Work out the finished part from the listing and answer in its coordinate system (mm). A direction names the side the tool comes from. Round coordinates to 2 decimals unless told otherwise and drop trailing zeros. Loops run counter-clockwise (first coordinate to the right, second up) from the corner with the lowest first, then second, coordinate; pieces in that order, holes last. Notation, with made-up numbers: (10.25, 57) -> (45.25, 57) arc R30 cw to (45.25, 81) -> close; hole circle Ø6 at (15, 60.5). An arc over 180 degrees is marked (long way). Write item = value, one per line. Start each with the question number.
```python
from build123d import *

# Parameters (mm, degrees)
BOSS_EXTRUDE1_DEPTH             = 50
BOSS_EXTRUDE2_START             = 13.15
BOSS_EXTRUDE2_DEPTH             = 13.15
BOSS_EXTRUDE3_DEPTH             = 21.75
BOSS_EXTRUDE3_DEPTH_BACK        = 63.15
CUT_EXTRUDE1_DEPTH              = 145.663436984
FILLET1_R                       = 3
CUT_EXTRUDE2_DEPTH              = 129.082637169
TAP_DRILL_FOR_M4X0_7_TAP1_D     = 3.3
TAP_DRILL_FOR_M4X0_7_TAP1_DEPTH = 10
TAP_DRILL_FOR_M4X0_7_TAP1_TIP   = 0.991420021


with BuildPart() as part:
    # Sketch1 → Boss-Extrude1 (new body)
    with BuildSketch(Plane.XY):
        with BuildLine():
            Line((36, 0), (63.5, 0))
            ThreePointArc((63.5, 0), (49.923691771, -39.241241061), (15, -61.702917273))
            Line((15, -61.702917273), (15, -32.726136344))
            ThreePointArc((15, -32.726136344), (30.298514815, -19.442222095), (36, 0))
        make_face()
    extrude(amount=BOSS_EXTRUDE1_DEPTH)

    # Sketch2 → Boss-Extrude2 (add)
    with BuildSketch(Plane(origin=(0, 0, 0), x_dir=(-1, 0, 0), z_dir=(0, 0, -1)).offset(BOSS_EXTRUDE2_START)):
        with BuildLine():
            Line((-45, 0), (-63.5, 0))
            ThreePointArc((-63.5, 0), (-49.923691771, -39.241241061), (-15, -61.702917273))
            Line((-15, -61.702917273), (-15, -42.426406871))
            ThreePointArc((-15, -42.426406871), (-36.742346142, -25.980762114), (-45, 0))
        make_face()
    extrude(amount=-BOSS_EXTRUDE2_DEPTH)

    # Sketch3 → Boss-Extrude3 (add, two sides: drawn at the far end of the back side and taken through both)
    with BuildSketch(Plane(origin=(0, 0, -13.15), x_dir=(-1, 0, 0), z_dir=(0, 0, -1)).offset(-BOSS_EXTRUDE3_DEPTH_BACK)):
        with BuildLine():
            Line((-63.5, 0), (-83.5, 0))
            ThreePointArc((-83.5, 0), (-64.127802083, -53.477799132), (-15, -82.141645954))
            Line((-15, -82.141645954), (-15, -61.702917273))
            ThreePointArc((-15, -61.702917273), (-49.923691771, -39.241241061), (-63.5, 0))
        make_face()
    extrude(amount=BOSS_EXTRUDE3_DEPTH + BOSS_EXTRUDE3_DEPTH_BACK)

    # Sketch4 → Cut-Extrude1 (cut, through all)
    with BuildSketch(Plane.XY.offset(50)):
        with BuildLine():
            Line((15, -32.726136344), (68.901001848, -47.16886626))
            ThreePointArc((68.901001848, -47.16886626), (45.449074332, -70.047352857), (15, -82.141645954))
            Line((15, -82.141645954), (15, -32.726136344))
        make_face()
    extrude(amount=-CUT_EXTRUDE1_DEPTH, mode=Mode.SUBTRACT)

    # Fillet1
    fillet1_edges = [part.edges().sort_by_distance(p)[0] for p in [
        (36, 0, 25),
        (15, -32.726136344, 25),
    ]]
    fillet(fillet1_edges, radius=FILLET1_R)

    # Sketch5 → Cut-Extrude2 (cut, through all)
    with BuildSketch(Plane.XY.offset(50)):
        with BuildLine():
            Line((83.5, 0), (68.901001848, -47.16886626))
            ThreePointArc((68.901001848, -47.16886626), (79.766796521, -24.688219313), (83.5, 0))
        make_face()
    extrude(amount=-CUT_EXTRUDE2_DEPTH, mode=Mode.SUBTRACT)

    # Tap Drill for M4x0.7 Tap1
    with Locations(Plane(origin=(76.200500924, -23.58443313, 0), x_dir=(0, 0, -1), z_dir=(0.9552909762953877, -0.29566729715781054, 0))):
        with Locations((-35, 15), (-35, -15), (-5, 15), (-5, -15)):
            Hole(TAP_DRILL_FOR_M4X0_7_TAP1_D / 2, depth=TAP_DRILL_FOR_M4X0_7_TAP1_DEPTH)
            with Locations((0, 0, -(TAP_DRILL_FOR_M4X0_7_TAP1_DEPTH + TAP_DRILL_FOR_M4X0_7_TAP1_TIP / 2))):  # 118° drill point
                Cone(0, TAP_DRILL_FOR_M4X0_7_TAP1_D / 2, TAP_DRILL_FOR_M4X0_7_TAP1_TIP, mode=Mode.SUBTRACT)


solid = part.part
```
Item 1: Find the intervals of material crossed by line 1 along Z through (x, y) = (61.5, -3); line 2 along Y through (x, z) = (49.5, 22.5); line 3 along X through (y, z) = (-28, 40), in increasing order. Write a range as [from, to].
Item 2: Section A-A (z = 8) is taken. Determine the outline of the cut face in (x, y).
Item 3: The mould has two halves that part along X. Classify faces 4 (the flat face through (61, 0, 18)), 5 (the cylindrical face through (66.94, -36.35, 33.35)), 6 (the cylindrical face through (59.388, -22.479, -23.873)): pulls with the +X half, pulls with the -X half, needs draft (parallel to the pull), parting line crosses it, or undercut.
Item 4: Section D-D (y = -22) is taken. Determine the outline of the cut face in (x, z).
Item 5: A tool of negligible diameter and unlimited length cuts with its end or side. For faces 1 (the cylindrical face through (40.134, -20.353, -6.667)), 2 (the cylindrical face through (31.261, -17.853, 24.65)), 3 (the conical face through (70.304, -6.044, 35.286)), from which of +Z, -Z, +X, -X, +Y, -Y can it reach the whole face along a straight path? Write none if from no direction.
Item 6: Flat-ended cylindrical pins translate along their axes: pin 1 (1.5 mm diameter, centred on x = 50, y = -15, fed in from -Z); pin 2 (6 mm diameter, centred on y = -38, z = 27.5, fed in from +X); pin 3 (3 mm diameter, centred on y = -26.5, z = -13.5, fed in from -X); pin 4 (11 mm diameter, centred on x = 53, y = -31, fed in from -Z). Find the tip coordinate at first contact, or state that the pin passes through.
Item 7: Section C-C (x = 31) is taken. Determine the outline of the cut face in (y, z), then the cut area to 3 significant figures.
Item 8: Section B-B (y = -31) is taken. Determine the outline of the cut face in (x, z), then the cut area to 3 significant figures.
Worked answers:
q1.line_1 = [-13.15, 50]
q1.line_2 = [-41.97, 0]
q1.line_3 = [22.63, 74.83]
q2.outline = (20.98, -29.25) arc R3 ccw to (21.95, -34.59) -> (68.9, -47.17) -> (83.5, 0) -> (38.88, 0) arc R3 ccw to (35.89, -2.77) arc R36 cw to start
q3.face_4 = needs draft
q3.face_5 = undercut
q3.face_6 = pulls with the -X half
q4.outline = (28.5, 0) -> (39.26, 0) -> (39.26, -13.15) -> (59.57, -13.15) -> (59.57, -34.9) -> (76.69, -34.9) -> (76.69, 50) -> (28.5, 50) -> close
q5.face_1 = -Z, -X, +Y
q5.face_2 = +Z, -Z, -X, +Y
q5.face_3 = none
q6.pin_1 = -13.15
q6.pin_2 = 72.67
q6.pin_3 = 35.26
q6.pin_4 = -34.9
q7.outline = (-37.01, -13.15) -> (-32.62, -13.15) -> (-32.62, 0) -> (-18.3, 0) -> (-18.3, 50) -> (-37.01, 50) -> close
q7.area = 993 mm2
q8.outline = (19.81, 0) -> (32.62, 0) -> (32.62, -13.15) -> (55.42, -13.15) -> (55.42, -34.9) -> (73.91, -34.9) -> (73.91, 50) -> (19.81, 50) -> close
q8.area = 3,650 mm2
